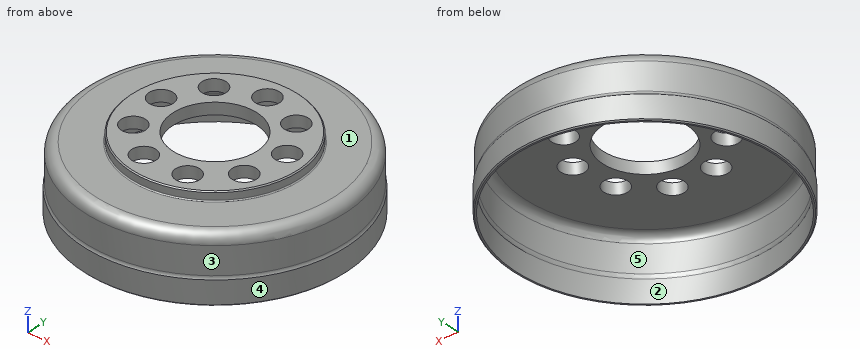
from build123d import *

# Parameters (mm, degrees)
SKETCH1_R           = 25
BOSS_EXTRUDE1_DEPTH = 4.5
SKETCH2_R           = 24.8
BOSS_EXTRUDE2_DEPTH = 7.8
FILLET1_R           = 2
FILLET2_R           = 1
SHELL1_T            = -0.5
CHAMFER1_SIZE       = 0.2
SKETCH3_R           = 16
BOSS_EXTRUDE3_DEPTH = 1.7
CHAMFER2_SIZE       = 0.2
FILLET3_R           = 0.2
SKETCH4_R           = 8
SKETCH4_R_2         = 2.3
CUT_EXTRUDE1_DEPTH  = 39.026306684


with BuildPart() as part:
    # Sketch1 → Boss-Extrude1 (new body)
    with BuildSketch(Plane.XY):
        Circle(SKETCH1_R)
    extrude(amount=BOSS_EXTRUDE1_DEPTH)

    # Sketch2 → Boss-Extrude2 (add)
    with BuildSketch(Plane.XY.offset(4.5)):
        Circle(SKETCH2_R)
    extrude(amount=BOSS_EXTRUDE2_DEPTH)

    # Fillet1
    fillet1_edges = [part.edges().sort_by_distance(p)[0] for p in [
        (-24.8, 0, 12.3),
    ]]
    fillet(fillet1_edges, radius=FILLET1_R)

    # Fillet2
    # the kernel refuses this fillet: 1 mm, written as the material it adds along each edge
    with BuildSketch(Plane(origin=(0, 0, 4.5), x_dir=(1, 0, 0), z_dir=(0, -1, 0))) as fillet2_piece_1:
        with BuildLine():
            CenterArc((25.8, 0.6), FILLET2_R, 180, 36.869897646)
            Line((25, 0), (24.984, -0.012))
            ThreePointArc((24.984, -0.012), (24.9, -0.02), (24.8, -0.02))
            Line((24.8, -0.02), (24.78, 0))
            Line((24.78, 0), (24.78, 0.6))
            Line((24.78, 0.6), (24.8, 0.6))
        make_face()
    revolve(axis=Axis((0, 0, 4.5), (0, 0, 1)))

    # Shell1
    shell1_openings = [part.faces().sort_by_distance(p)[0] for p in [
        (0, 0, 0),
    ]]
    offset(amount=SHELL1_T, openings=shell1_openings, kind=Kind.INTERSECTION)

    # Chamfer1
    chamfer1_edges = [part.edges().sort_by_distance(p)[0] for p in [
        (-25, 0, 0),
    ]]
    chamfer(chamfer1_edges, length=CHAMFER1_SIZE)

    # Sketch3 → Boss-Extrude3 (add)
    with BuildSketch(Plane.XY.offset(12.3)):
        Circle(SKETCH3_R)
    extrude(amount=BOSS_EXTRUDE3_DEPTH)

    # Chamfer2
    chamfer2_edges = [part.edges().sort_by_distance(p)[0] for p in [
        (-16, 0, 14),
    ]]
    chamfer(chamfer2_edges, length=CHAMFER2_SIZE)

    # Fillet3
    fillet3_edges = [part.edges().sort_by_distance(p)[0] for p in [
        (-16, 0, 12.3),
    ]]
    fillet(fillet3_edges, radius=FILLET3_R)

    # Sketch4 → Cut-Extrude1 (cut, through all)
    with BuildSketch(Plane.XY.offset(14)):
        Circle(SKETCH4_R)
        with Locations((0, 12.024661136)):
            Circle(SKETCH4_R_2)
        with Locations((7.729303189, 9.211424844)):
            Circle(SKETCH4_R_2)
        with Locations((11.841979514, 2.088060493)):
            Circle(SKETCH4_R_2)
        with Locations((10.413662016, -6.012330568)):
            Circle(SKETCH4_R_2)
        with Locations((4.112676325, -11.299485337)):
            Circle(SKETCH4_R_2)
        with Locations((-4.112676325, -11.299485337)):
            Circle(SKETCH4_R_2)
        with Locations((-10.413662016, -6.012330568)):
            Circle(SKETCH4_R_2)
        with Locations((-11.841979514, 2.088060493)):
            Circle(SKETCH4_R_2)
        with Locations((-7.729303189, 9.211424844)):
            Circle(SKETCH4_R_2)
    extrude(amount=-CUT_EXTRUDE1_DEPTH, mode=Mode.SUBTRACT)


solid = part.part
The model under review builds one solid part; all positions refer to its coordinate system, in mm. Face numbers are marked on the shaded views. A direction names the side the tool comes from. Round coordinates to 2 decimals unless told otherwise and drop trailing zeros. Loops run counter-clockwise (first coordinate to the right, second up) from the corner with the lowest first, then second, coordinate; pieces in that order, holes last. Notation, with made-up numbers: M 59,53 L 64,53 A15 cw 64,79 Z; hole C 39.5,-4 d6. An arc over 180 degrees is marked long. Answer as a JSON object with one key per item and string values.
Item 1: Tool access review of the marked faces 4 and 5: name each direction out of +Z, -Z, +X, -X, +Y, -Y from which nothing blocks a thin tool from reaching the whole face with its end or side.
Check sheet entries:
{"face 4": "+Z, -Z", "face 5": "-Z"}
Item 2: We need section A-A, the plane x = 0. State how many separate pieces and enclosed holes the cut face has, and give its area (3 significant figures).
Check sheet entries:
{"separate pieces": "3", "enclosed holes": "0", "area": "44.9 mm2"}
Item 3: For line 1 along Y through (x, z) = (0, 1); line 2 along Y through (x, z) = (12, 13.25); line 3 along Z through (x, y) = (-10.5, 19), list the stretches that pass through material, from the lowest coordinate up.
Check sheet entries:
{"line 1": "-25 to -24.5, 24.5 to 25", "line 2": "-10.58 to -7.68, -4.35 to -0.21, 4.38 to 10.58", "line 3": "11.8 to 12.3"}
Item 4: The part is to be moulded in two halves that separate along Y. For the marked faces 1, 2 and 3, say which applies: +Y half, -Y half, draft (parallel to the pull), parting line (faces both ways), or undercut.
Check sheet entries:
{"face 1": "draft", "face 2": "undercut", "face 3": "parting line"}
Item 5: We need section B-B, the plane z = 1.25. State the section outline as (x, y) points.
Check sheet entries:
{"outline": "C 0,0 d50; hole C 0,0 d49"}
Item 6: Clearance check with flat-ended pins moving along their axes: P1, Ø1, axis at x = 15, z = 11.5, coming from the +Y side; P2, Ø4, axis at y = -20, z = 11, coming from the -X side; P3, Ø7.5, axis at x = 11.84, y = 2.09, coming from the -Z side. State where each tip first meets the part, or that it passes through.
Check sheet entries:
{"P1": "y = 19.78", "P2": "x = -16.98", "P3": "z = 11.8"}
